Can you work these out from the model? Positions are in its coordinate system, mm. A direction names the side the tool comes from. Round coordinates to 2 decimals unless told otherwise and drop trailing zeros. Loops run counter-clockwise (first coordinate to the right, second up) from the corner with the lowest first, then second, coordinate; pieces in that order, holes last. Notation, with made-up numbers: M -28,51.25 L 26,51.25 A21 ccw 26,88.25 Z; hole C -31,36.25 d5. An arc over 180 degrees is marked long. Return JSON: item names as keys, results as strings.
```python
from build123d import *

# Parameters (mm, degrees)
SKETCH1_R           = 15.875
BOSS_EXTRUDE1_DEPTH = 15
SKETCH2_R           = 25.391657194
SKETCH2_R_2         = 7.9375
CUT_EXTRUDE1_DEPTH  = 10
SKETCH3_R           = 3.96875
CUT_EXTRUDE2_DEPTH  = 28.000578698
BOSS_EXTRUDE2_START = 3
SKETCH4_R           = 4.699
SKETCH4_R_2         = 3.96875
BOSS_EXTRUDE2_DEPTH = 3
SKETCH5_R           = 1.5875
CUT_EXTRUDE3_DEPTH  = 28.000578698
SKETCH6_R           = 1.27
CUT_EXTRUDE4_DEPTH  = 28.000578698
SKETCH7_R           = 1.27
CUT_EXTRUDE5_DEPTH  = 28.000578753


with BuildPart() as part:
    # Sketch1 → Boss-Extrude1 (new body)
    with BuildSketch(Plane.XY):
        Circle(SKETCH1_R)
    extrude(amount=BOSS_EXTRUDE1_DEPTH)

    # Sketch2 → Cut-Extrude1 (cut)
    with BuildSketch(Plane.XY.offset(15)):
        Circle(SKETCH2_R)
        Circle(SKETCH2_R_2, mode=Mode.SUBTRACT)
    extrude(amount=-CUT_EXTRUDE1_DEPTH, mode=Mode.SUBTRACT)

    # Sketch3 → Cut-Extrude2 (cut, through all)
    with BuildSketch(Plane(origin=(0, 0, 0), x_dir=(-1, 0, 0), z_dir=(0, 0, -1))):
        Circle(SKETCH3_R)
    extrude(amount=-CUT_EXTRUDE2_DEPTH, mode=Mode.SUBTRACT)

    # Sketch4 → Boss-Extrude2 (add)
    with BuildSketch(Plane(origin=(0, 0, 0), x_dir=(-1, 0, 0), z_dir=(0, 0, -1)).offset(BOSS_EXTRUDE2_START)):
        with Locations(Location((0, 0, 0), (0, 0, 180))):
            Circle(SKETCH4_R)
        Circle(SKETCH4_R_2, mode=Mode.SUBTRACT)
    extrude(amount=-BOSS_EXTRUDE2_DEPTH)

    # Sketch5 → Cut-Extrude3 (cut, through all)
    with BuildSketch(Plane(origin=(0, 0, 0), x_dir=(-1, 0, 0), z_dir=(0, 0, -1))):
        with Locations((0, 11)):
            Circle(SKETCH5_R)
        with Locations((9.526779442, 5.500866025)):
            Circle(SKETCH5_R)
        with Locations((9.527779442, -5.499133975)):
            Circle(SKETCH5_R)
        with Locations((0.002, -11)):
            Circle(SKETCH5_R)
        with Locations((-9.524779442, -5.500866025)):
            Circle(SKETCH5_R)
        with Locations((-9.525779442, 5.499133975)):
            Circle(SKETCH5_R)
    extrude(amount=-CUT_EXTRUDE3_DEPTH, mode=Mode.SUBTRACT)

    # Sketch6 → Cut-Extrude4 (cut, through all)
    with BuildSketch(Plane(origin=(0, 0, 0), x_dir=(1, 0, 0), z_dir=(0, 1, 0))):
        with Locations(Location((0, -10, 0), (0, 0, 90))):
            Circle(SKETCH6_R)
    extrude(amount=CUT_EXTRUDE4_DEPTH, mode=Mode.SUBTRACT)

    # Sketch7 → Cut-Extrude5 (cut, through all)
    with BuildSketch(Plane(origin=(0, 0, 0), x_dir=(0, 0, -1), z_dir=(1, 0, 0))):
        with Locations(Location((-10, 0, 0), (0, 0, 180))):
            Circle(SKETCH7_R)
    extrude(amount=CUT_EXTRUDE5_DEPTH, mode=Mode.SUBTRACT)


solid = part.part
```
Q1. On a 3-axis mill with a long thin cutter (end or side, diameter ignored), from which of +Z, -Z, +X, -X, +Y, -Y can I reach the whole of each face in a straight line? I mean faces 1 (the cylindrical face through (5.82, 0.49, 11.17)), 2 (the cylindrical face through (-1.72, -7.75, 10.07)), 3 (the flat face through (-4, -3, 0)). Say none if no direction works.
Results:
{"face 1": "+X", "face 2": "+Z", "face 3": "-Z"}
Q2. If I drill on line 1 along Y through (x, z) = (0, 3.3) (1 decimal); line 2 along Y through (x, z) = (-10.5, 4); line 3 along Y through (x, z) = (0.5, -1.5), over which ranges is the centre line in solid material (lowest first)?
Results:
{"line 1": "y = -15.9 to -12.6, -9.4 to -4, 4 to 9.4, 12.6 to 15.9", "line 2": "y = -11.91 to -6.75, -4.24 to 4.25, 6.76 to 11.91", "line 3": "y = -4.67 to -3.94, 3.94 to 4.67"}
Q3. Suppose I cut it at A-A, the plane x = 0. Please give me the cut outline in (y, z) (1 decimal).
Results:
{"outline": "M -15.9,0 L -12.6,0 L -12.6,5 L -15.9,5 Z; M -9.4,0 L -4.7,0 L -4.7,-3 L -4,-3 L -4,15 L -7.9,15 L -7.9,5 L -9.4,5 Z; M 4,-3 L 4.7,-3 L 4.7,0 L 9.4,0 L 9.4,5 L 7.9,5 L 7.9,8.7 L 4,8.7 Z; M 4,11.3 L 7.9,11.3 L 7.9,15 L 4,15 Z; M 12.6,0 L 15.9,0 L 15.9,5 L 12.6,5 Z"}
Q4. Suppose I cut it at B-B, the plane y = 0. Please give me the cut outline in (x, z) (1 decimal).
Results:
{"outline": "M -15.9,0 L -4.7,0 L -4.7,-3 L -4,-3 L -4,15 L -7.9,15 L -7.9,5 L -15.9,5 Z; M 4,-3 L 4.7,-3 L 4.7,0 L 15.9,0 L 15.9,5 L 7.9,5 L 7.9,8.7 L 4,8.7 Z; M 4,11.3 L 7.9,11.3 L 7.9,15 L 4,15 Z"}
Q5. I'm going to push flat-ended pins straight in: pin 1 Ø4 at (x, z) = (8, 10.5) entering from -Y; pin 2 Ø4 at (x, y) = (-7.5, -6.5) entering from -Z; pin 3 Ø1.9 at (x, y) = (9.53, 5.5) entering from +Z; pin 4 Ø2.5 at (x, z) = (0, 10) entering from -Y. Where does each tip first touch, or does it pass through?
Results:
{"pin 1": "stops at y = -5.2", "pin 2": "stops at z = 0", "pin 3": "passes through", "pin 4": "stops at y = -7.94"}
Q6. Suppose I cut it at C-C, the plane z = 10. Please give me the cut outline in (x, y) (1 decimal), plus the area to 3 significant figures.
Results:
{"outline": "M -1.3,3.8 L -1.3,7.8 A7.9 ccw long 7.8,-1.3 L 3.8,-1.3 A4 cw long Z; M 1.3,3.8 A4 cw 3.8,1.3 L 7.8,1.3 A7.9 ccw 1.3,7.8 Z", "area": "128 mm2"}
Q7. Suppose I cut it at D-D, the plane z = 1.25. State how many separate pieces and enclosed holes the cut face has, plus the area to 3 significant figures.
Results:
{"separate pieces": "1", "enclosed holes": "7", "area": "695 mm2"}
Q8. Thinking about a two-plate mould opening in Z: for faces 4 (the cylindrical face through (0.49, 5.82, 8.83)), 5 (the flat face through (-7.3, 3.8, 5)), 6 (the cylindrical face through (0.205, -9.426, 2.465)), which applies, pulls with the +Z half, pulls with the -Z half, needs draft (parallel to the pull), parting line crosses it, or undercut?
Results:
{"face 4": "undercut", "face 5": "pulls with the +Z half", "face 6": "needs draft"}
